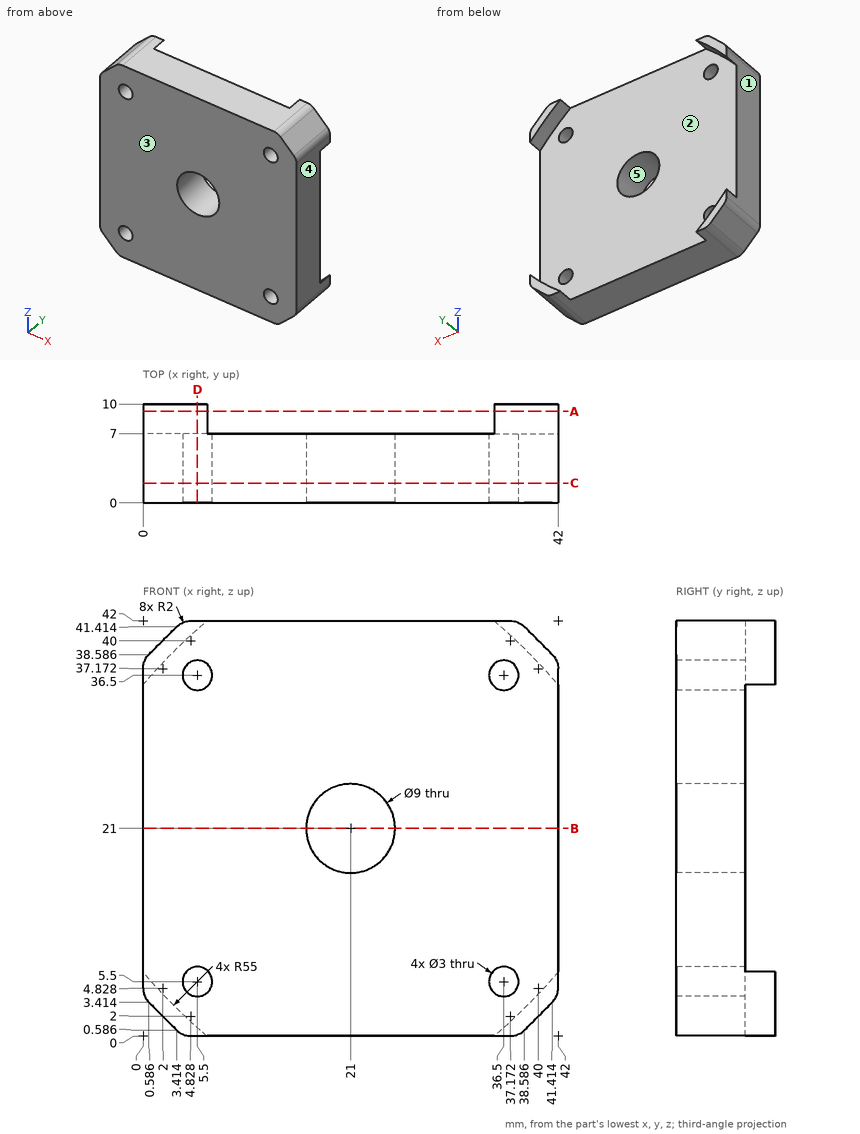
For this review, use the dimensioned drawing (mm, ordinates from the lowest corner) and the shaded views. A direction names the side the tool comes from. Round coordinates to 2 decimals unless told otherwise and drop trailing zeros. Write each loop counter-clockwise with the first axis right and the second up, starting at its lowest first coordinate (ties: lowest second). Pieces come first, ordered by that corner, then holes. Notation, with made-up numbers: M 51,-19 L 62,-19 A22 ccw 62,12 Z; hole C -14.5,61 d9. An arc over 180 degrees is marked long. Answer as CSV lines item,"result". Start each with the question number.
Q1. Tool access review of the marked faces 1 and 2: name each direction out of +Z, -Z, +X, -X, +Y, -Y from which nothing blocks a thin tool from reaching the whole face with its end or side.
Q2. Wall thickness on line 1 along Z through (x, y) = (36.5, 4); line 2 along Z through (x, y) = (21, 1.5); line 3 along Y through (x, z) = (13, 36.5): over which ranges is each line inside the solid? List them lowest first.
Q3. Consider section B-B, the plane z = 21. Give the boundary of the cut face in (x, y), then the cut area to 3 significant figures.
Q4. Clearance check with flat-ended pins moving along their axes: P1, Ø1, axis at x = 29, z = 25.5, coming from the +Y side; P2, Ø1.8, axis at x = 36.5, z = 36.5, coming from the +Y side (3 decimals). State where each tip first meets the part, or that it passes through.
Q5. The part is to be moulded in two halves that separate along X. For the marked faces 3, 4 and 5, say which applies: +X half, -X half, draft (parallel to the pull), parting line (faces both ways), or undercut.
Q6. Consider section D-D, the plane x = 5.5. Give the boundary of the cut face in (y, z).
Q7. Consider section A-A, the plane y = 9.25. Give the boundary of the cut face in (x, z) (1 decimal).
Q8. Consider section C-C, the plane y = 2. Give the boundary of the cut face in (x, z) (1 decimal).
Result set:
1,face 1,"+Z, -Z, -X, +Y, -Y"
1,face 2,"+Y"
2,line 1,"z = 0 to 4, 7 to 35, 38 to 42"
2,line 2,"z = 0 to 16.5, 25.5 to 42"
2,line 3,"y = 0 to 7"
3,outline,"M 0,0 L 16.5,0 L 16.5,7 L 0,7 Z; M 25.5,0 L 42,0 L 42,7 L 25.5,7 Z"
3,area,"231 mm²"
4,P1,"stops at y = 7"
4,P2,"passes through"
5,face 3,"draft"
5,face 4,"+X half"
5,face 5,"undercut"
6,outline,"M 0,0 L 10,0 L 10,0.86 L 7,0.86 L 7,4 L 0,4 Z; M 0,7 L 7,7 L 7,35 L 0,35 Z; M 0,38 L 7,38 L 7,41.14 L 10,41.14 L 10,42 L 0,42 Z"
7,outline,"M 0,4.8 A2 ccw 0.6,3.4 L 3.4,0.6 A2 ccw 4.8,0 L 6.5,0 A55 cw 0,6.5 Z; M 0,35.5 A55 cw 6.5,42 L 4.8,42 A2 ccw 3.4,41.4 L 0.6,38.6 A2 ccw 0,37.2 Z; M 35.5,0 L 37.2,0 A2 ccw 38.6,0.6 L 41.4,3.4 A2 ccw 42,4.8 L 42,6.5 A55 cw Z; M 35.5,42 A55 cw 42,35.5 L 42,37.2 A2 ccw 41.4,38.6 L 38.6,41.4 A2 ccw 37.2,42 Z"
8,outline,"M 0,4.8 A2 ccw 0.6,3.4 L 3.4,0.6 A2 ccw 4.8,0 L 37.2,0 A2 ccw 38.6,0.6 L 41.4,3.4 A2 ccw 42,4.8 L 42,37.2 A2 ccw 41.4,38.6 L 38.6,41.4 A2 ccw 37.2,42 L 4.8,42 A2 ccw 3.4,41.4 L 0.6,38.6 A2 ccw 0,37.2 Z; hole C 5.5,5.5 d3; hole C 5.5,36.5 d3; hole C 21,21 d9; hole C 36.5,5.5 d3; hole C 36.5,36.5 d3"
